The model under review builds one solid part; all positions refer to its coordinate system, in mm. Coordinates: 2 decimals unless noted, no trailing zeros. Order: outer loops, then holes, each group sorted by start corner. A loop starts at its lowest first (then second) coordinate and runs counter-clockwise, first axis right, second up. Notation, with made-up numbers: M 1.25,22 L 60.25,22 A32 ccw 60.25,50 Z; hole C -27,77.5 d10. An arc over 180 degrees is marked long. Answer in a Markdown table with one row per item.
from build123d import *

# Parameters (mm, degrees)
SKETCH1_R           = 132.334
BOSS_EXTRUDE1_DEPTH = 1.524


with BuildPart() as part:
    # Sketch1 → Boss-Extrude1 (new body)
    with BuildSketch(Plane(origin=(0, 0, 0), x_dir=(1, 0, 0), z_dir=(0, 1, 0))):
        with Locations(Location((0, 0, 0), (0, 0, 90))):
            Circle(SKETCH1_R)
        with BuildLine():
            ThreePointArc((-92.388062371, 85.65287028), (-116.394039024, 48.211989543), (-125.893950807, 4.7625))
            Line((-125.893950807, 4.7625), (-11.497692091, 4.7625))
            Line((-11.497692091, 4.7625), (-92.388062371, 85.65287028))
        make_face(mode=Mode.SUBTRACT)
        with BuildLine():
            ThreePointArc((-125.893950807, -4.7625), (-116.394039024, -48.211989543), (-92.388062371, -85.65287028))
            Line((-92.388062371, -85.65287028), (-11.497692091, -4.7625))
            Line((-11.497692091, -4.7625), (-125.893950807, -4.7625))
        make_face(mode=Mode.SUBTRACT)
        with BuildLine():
            ThreePointArc((-85.65287028, -92.388062371), (-48.211989543, -116.394039024), (-4.7625, -125.893950807))
            Line((-4.7625, -125.893950807), (-4.7625, -11.497692091))
            Line((-4.7625, -11.497692091), (-85.65287028, -92.388062371))
        make_face(mode=Mode.SUBTRACT)
        with BuildLine():
            ThreePointArc((4.7625, -125.893950807), (48.211989543, -116.394039024), (85.65287028, -92.388062371))
            Line((85.65287028, -92.388062371), (4.7625, -11.497692091))
            Line((4.7625, -11.497692091), (4.7625, -125.893950807))
        make_face(mode=Mode.SUBTRACT)
        with BuildLine():
            ThreePointArc((92.388062371, -85.65287028), (116.394039024, -48.211989543), (125.893950807, -4.7625))
            Line((125.893950807, -4.7625), (11.497692091, -4.7625))
            Line((11.497692091, -4.7625), (92.388062371, -85.65287028))
        make_face(mode=Mode.SUBTRACT)
        with BuildLine():
            ThreePointArc((125.893950807, 4.7625), (116.394039024, 48.211989543), (92.388062371, 85.65287028))
            Line((92.388062371, 85.65287028), (11.497692091, 4.7625))
            Line((11.497692091, 4.7625), (125.893950807, 4.7625))
        make_face(mode=Mode.SUBTRACT)
        with BuildLine():
            ThreePointArc((85.65287028, 92.388062371), (48.211989543, 116.394039024), (4.7625, 125.893950807))
            Line((4.7625, 125.893950807), (4.7625, 11.497692091))
            Line((4.7625, 11.497692091), (85.65287028, 92.388062371))
        make_face(mode=Mode.SUBTRACT)
        with BuildLine():
            ThreePointArc((-4.7625, 125.893950807), (-48.211989543, 116.394039024), (-85.65287028, 92.388062371))
            Line((-85.65287028, 92.388062371), (-4.7625, 11.497692091))
            Line((-4.7625, 11.497692091), (-4.7625, 125.893950807))
        make_face(mode=Mode.SUBTRACT)
    extrude(amount=BOSS_EXTRUDE1_DEPTH)


solid = part.part
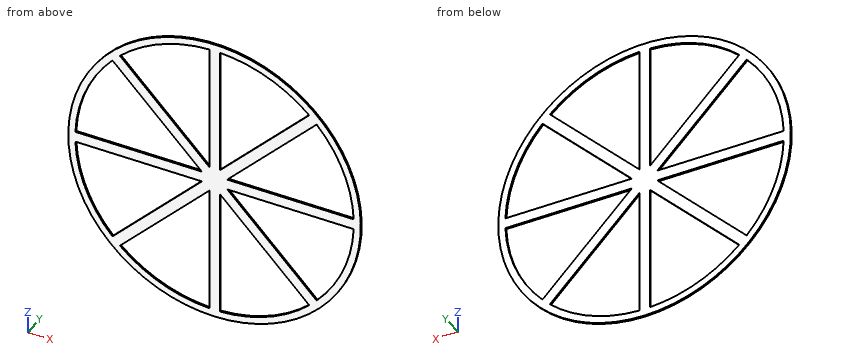
(1) Take a section at D-D (z = -99.5). Write out the cut boundary in (x, y).
Report:
| item | result |
|---|---|
| outline | M -87.25,0 L -77.28,0 L -77.28,1.52 L -87.25,1.52 Z; M -4.76,0 L 4.76,0 L 4.76,1.52 L -4.76,1.52 Z; M 77.28,0 L 87.25,0 L 87.25,1.52 L 77.28,1.52 Z |
(2) Take a section at C-C (x = -53). Write out the cut boundary in (y, z), then the cut area to 3 significant figures.
Report:
| item | result |
|---|---|
| outline | M 0,-121.26 L 1.52,-121.26 L 1.52,-114.29 L 0,-114.29 Z; M 0,-59.74 L 1.52,-59.74 L 1.52,-46.26 L 0,-46.26 Z; M 0,-4.76 L 1.52,-4.76 L 1.52,4.76 L 0,4.76 Z; M 0,46.26 L 1.52,46.26 L 1.52,59.74 L 0,59.74 Z; M 0,114.29 L 1.52,114.29 L 1.52,121.26 L 0,121.26 Z |
| area | 76.8 mm^2 |
(3) Take a section at A-A (y = 1). State how many separate pieces and enclosed holes the cut face has, then the cut area to 3 significant figures.
Report:
| item | result |
|---|---|
| separate pieces | 1 |
| enclosed holes | 8 |
| area | 14,300 mm^2 |
(4) Insertion check: P1, Ø0.8, axis at x = -89.5, y = 1, coming from the -Z side; P2, Ø0.8, axis at x = 57, y = 1, coming from the +Z side. Each pin has a flat end and moves straight along its axis. Give the tip position at first contact, or say it passes through.
Report:
| item | result |
|---|---|
| P1 | z = -97.84 |
| P2 | z = 119.62 |
(5) Take a section at B-B (z = 47.5). Write out the cut boundary in (x, y), then the cut area to 3 significant figures.
Report:
| item | result |
|---|---|
| outline | M -123.52,0 L -116.69,0 L -116.69,1.52 L -123.52,1.52 Z; M -54.24,0 L -40.76,0 L -40.76,1.52 L -54.24,1.52 Z; M -4.76,0 L 4.76,0 L 4.76,1.52 L -4.76,1.52 Z; M 40.76,0 L 54.24,0 L 54.24,1.52 L 40.76,1.52 Z; M 116.69,0 L 123.52,0 L 123.52,1.52 L 116.69,1.52 Z |
| area | 76.4 mm^2 |
(6) To check wall thickness, follow line 1 (X direction, y = 1.4, z = -20); line 2 (Z direction, x = 14, y = 1.45); line 3 (X direction, y = 0.35, z = -73). State the ranges of each line that lie inside material, in increasing order. Write a range as [from, to].
Report:
| item | result |
|---|---|
| line 1 | [-130.81, -124.39], [-26.74, -13.26], [-4.76, 4.76], [13.26, 26.74], [124.39, 130.81] |
| line 2 | [-131.59, -125.2], [-20.74, -7.26], [-4.76, 4.76], [7.26, 20.74], [125.2, 131.59] |
| line 3 | [-110.38, -102.68], [-79.74, -66.26], [-4.76, 4.76], [66.26, 79.74], [102.68, 110.38] |
